The model under review builds one solid part; all positions refer to its coordinate system, in mm. A direction names the side the tool comes from. Give positions to 0.01 mm unless a question says otherwise; leave off trailing zeros. Order: outer loops, then holes, each group sorted by start corner. A loop starts at its lowest first (then second) coordinate and runs counter-clockwise, first axis right, second up. Notation, with made-up numbers: (77.25, 28) - (106.25, 28) arc R13 ccw to (106.25, 49) - close; hole circle Ø7 at (-27.5, 88.5). An arc over 180 degrees is marked (long way). Put each result on its own line as item: value.
Autodesk Inventor part; units mm, degrees
ref_plane "YZ Plane" through (0, 0, 0) normal (1, 0, 0) x (0, 1, 0)
ref_plane "XZ Plane" through (0, 0, 0) normal (0, 1, 0) x (-1, 0, 0)
ref_plane "XY Plane" through (0, 0, 0) normal (0, 0, 1) x (1, 0, 0)
sketch "Sketch1" plane through (0, 0, 0) normal (0, 1, 0) x (-1, 0, 0)
  line L0 (0, 0) -> (-127, 0)
  line L1 (-127, 0) -> (-127, -122.428)
  line L2 (-127, -122.428) -> (0, -122.428)
  line L3 (0, -122.428) -> (0, 0)
  line L4 (0, 0) -> (-47.752, 0)
  line L5 (-47.752, 0) -> (-47.752, -53.34)
  line L6 (-47.752, -53.34) -> (0, -53.34)
  line L7 (0, -53.34) -> (0, 0)
  line L8 (-127, -122.428) -> (-50.8, -122.428)
  line L9 (-50.8, -122.428) -> (-50.8, 0)
  line L10 (-50.8, 0) -> (-127, 0)
  line L11 (-127, 0) -> (-127, -122.428)
  line L12 (-47.752, -53.34) -> (-50.8, -53.34)
  line L13 (-50.8, -53.34) -> (-50.8, 0)
  line L14 (-50.8, 0) -> (-47.752, 0)
  line L15 (-47.752, 0) -> (-47.752, -53.34)
  circle A0 centre (-11.938, -11.176) radius 3.175
  circle A1 centre (-35.814, -33.528) radius 3.175
  circle A2 centre (-11.938, -111.252) radius 3.175
  circle A3 centre (-35.814, -88.9) radius 3.175
  circle A4 centre (-73.914, -11.684) radius 1.5875
  circle A5 centre (-73.914, -41.656) radius 1.5875
  circle A6 centre (-103.886, -41.656) radius 1.5875
  circle A7 centre (-103.886, -11.684) radius 1.5875
  circle A8 centre (-88.9, -26.67) radius 4.953
  dimension "d0" = 127
  dimension "d1" = 122.428
  dimension "d2" = 47.752
  dimension "d3" = 53.34
  dimension "d4" = 76.2
  dimension "d5" = 11.176
  dimension "d6" = 22.352
  dimension "d7" = 38.1
  dimension "d8" = 14.986
  dimension "d9" = 14.986
  dimension "d10" = 14.986
  dimension "d11" = 14.986
  dimension "d12" = 6.35
  dimension "d13" = 6.35
  dimension "d14" = 6.35
  dimension "d15" = 6.35
  dimension "d16" = 3.175
  dimension "d17" = 3.175
  dimension "d18" = 3.175
  dimension "d19" = 3.175
  dimension "d20" = 9.906
  dimension "d21" = 11.176
  dimension "d22" = 11.938
  dimension "d23" = 23.876
  dimension "d24" = 22.352
  dimension "d25" = 11.938
  dimension "d26" = 11.938
  dimension "d27" = 23.876
extrude "Extrusion1" add sketch "Sketch1" along normal blind 3.175 contours L3 L6 L5 L0 | L3 L2 L9 L12 L6 | L9 L2 L1 L0
fillet "Fillet1" radius 19.05 3 edges at (127, 1.5875, 0) (50.8, 1.5875, 0) (127, 1.5875, -122.428)
properties part number "ARMS MOUNTING BRACKET"
(1) For faces 5 (the flat face through (50.8, 2, -36)), 6 (the cylindrical face through (105.472, 1.565, -11.754)), list the 3-axis set-ups (+Z, -Z, +X, -X, +Y, -Y) from which the entire face can be reached by the end or side of a thin tool; tool diameter is ignored.
The answers:
face 5: +Z, +Y, -Y
face 6: +Y, -Y
(2) Wall thickness on L1, parallel to X at y = 2.6, z = -36; L2, parallel to X at y = 1.4, z = -47.5; L3, parallel to Z at x = 73.5, y = 1.5: over which ranges is each line inside the solid? List them lowest first.
The answers:
L1: 0 to 33.82, 37.81 to 47.75, 50.8 to 127
L2: 0 to 47.75, 50.8 to 127
L3: -122.43 to -43.19, -40.12 to -13.22, -10.15 to 0
(3) Take a section at D-D, the plane x = 118. Write out the cut boundary in (y, z) (3 decimals), then the cut area to 3 significant figures.
The answers:
outline: (0, -119.561) - (3.175, -119.561) - (3.175, -2.867) - (0, -2.867) - close
area: 371 mm^2
(4) Take a section at A-A, the plane z = -38.5. Write out the cut boundary in (x, y) (3 decimals).
The answers:
outline: (0, 0) - (47.752, 0) - (47.752, 3.175) - (0, 3.175) - close; (50.8, 0) - (127, 0) - (127, 3.175) - (50.8, 3.175) - close
(5) Clearance check with flat-ended pins moving along their axes: pin 1 Ø5 at (x, z) = (103.886, -11.684) entering from -Y; pin 2 Ø1.5 at (x, y) = (49, 2.5) entering from +Z. State where each tip first meets the part, or that it passes through.
The answers:
pin 1: y = 0
pin 2: z = -53.34
(6) Take a section at C-C, the plane x = 35.5. Write out the cut boundary in (y, z) (3 decimals), then the cut area to 3 significant figures.
The answers:
outline: (0, -122.428) - (3.175, -122.428) - (3.175, -92.059) - (0, -92.059) - close; (0, -85.741) - (3.175, -85.741) - (3.175, -36.687) - (0, -36.687) - close; (0, -30.369) - (3.175, -30.369) - (3.175, 0) - (0, 0) - close
area: 349 mm^2
(7) Take a section at B-B, the plane x = 88.9. Write out the cut boundary in (y, z) (3 decimals).
The answers:
outline: (0, -122.428) - (3.175, -122.428) - (3.175, -31.623) - (0, -31.623) - close; (0, -21.717) - (3.175, -21.717) - (3.175, 0) - (0, 0) - close
(8) The part is to be moulded in two halves that separate along X. For faces 1 (the flat face through (127, 2, -61)), 2 (the flat face through (49, 2, -53.34)), 3 (the flat face through (55, 2, -122.428)), 4 (the flat face through (0, 2, -62)), say which applies: pulls with the +X half, pulls with the -X half, needs draft (parallel to the pull), parting line crosses it, or undercut.
The answers:
face 1: pulls with the +X half
face 2: undercut
face 3: needs draft
face 4: pulls with the -X half
